from build123d import *

# Parameters (mm, degrees)
F2_R     = 7.5
F3_DEPTH = 40
F4_R     = 3
F5_DEPTH = 25


with BuildPart() as f1:
    # F0 (on Front) → F1 (revolve)
    with BuildSketch(Plane.XZ):
        Polygon((-78.328885, 0), (-47.328885, 0), (-47.328885, 19.231284), (-58.328885, 19.231284), (-58.328885, 17.231284), (-60.328885, 17.231284), (-60.328885, 19.231284), (-62.328885, 19.231284), (-62.328885, 17.231284), (-64.328885, 17.231284), (-64.328885, 19.231284), (-66.328885, 19.231284), (-66.328885, 17.231284), (-68.328885, 17.231284), (-68.328885, 19.231284), (-78.328885, 19.231284), align=None)
    revolve(axis=Axis((-39.164443, 0, 0), (-1, 0, 0)))

    # F2 (on face) → F3 (cut)
    with BuildSketch(Plane(origin=(-78.328885, 0, 0), x_dir=(0, -1, 0), z_dir=(-1, 0, 0))):
        Circle(F2_R)
    extrude(amount=-F3_DEPTH, mode=Mode.SUBTRACT)

    # F4 (on Top) → F5 (cut)
    with BuildSketch(Plane.XY):
        with Locations((-52.106317, 0)):
            Circle(F4_R)
    extrude(amount=F5_DEPTH, mode=Mode.SUBTRACT)


solid = f1.part
Design review of the part built by this model. Coordinates are the model's own, in mm. A direction names the side the tool comes from. Round coordinates to 2 decimals unless told otherwise and drop trailing zeros. Write each loop counter-clockwise with the first axis right and the second up, starting at its lowest first coordinate (ties: lowest second). Pieces come first, ordered by that corner, then holes. Notation, with made-up numbers: (17.5, 26.25) -> (37.5, 26.25) arc R9 ccw to (37.5, 32.25) -> close; hole circle Ø6 at (-2, 5.25). An arc over 180 degrees is marked (long way). One line per item, written item: value. Start each with the question number.
Q1. Add section D-D (x = -67). Give the boundary of the cut face in (y, z).
Q2. The part is to be moulded in two halves that separate along Y. For faces 1 (the face through (-61.343, -11.702, -15.261)), 2 (the face through (-49.245, 0.901, 12.966)), 3 (the face through (-66.329, 7, -16)), 4 (the face through (-63.05, 1.63, -7.32)), say which applies: pulls with the +Y half, pulls with the -Y half, needs draft (parallel to the pull), parting line crosses it, or undercut.
Q3. To check wall thickness, follow probe 1 along X at (y, z) = (0, 10); probe 2 along X at (y, z) = (-11, -15.5); probe 3 along Y at (x, z) = (-48.5, 6). State the ranges of each line that lie inside material, in increasing order.
Q4. Insertion check: P1, Ø12, axis at x = -72, y = 12.5, coming from the +Z side; P2, Ø6, axis at x = -68.5, z = -8, coming from the +Y side; P3, Ø12, axis at x = -74.5, z = 11, coming from the -Y side; P4, Ø17, axis at y = 0, z = 0, coming from the -X side. Each pin has a flat end and moves straight along its axis. Give the tip position at first contact, or say it passes through.
Q5. Tool access review of faces 5 (the face through (-73.399, -11.702, -15.261)), 6 (the face through (-62.329, 7, -16)): name each direction out of +Z, -Z, +X, -X, +Y, -Y from which nothing blocks a thin tool from reaching the whole face with its end or side.
Response:
1. outline: circle Ø34.46 at (0, 0); hole circle Ø15 at (0, 0)
2. face 1: parting line crosses it
2. face 2: undercut
2. face 3: needs draft
2. face 4: undercut
3. probe 1: x = -78.33 to -55.11, -49.11 to -47.33
3. probe 2: x = -78.33 to -68.33, -66.33 to -64.33, -62.33 to -60.33, -58.33 to -47.33
3. probe 3: y = -18.27 to -4.5, 4.5 to 18.27
4. P1: stops at z = 18.1
4. P2: stops at y = 18.57
4. P3: stops at y = -18.57
4. P4: stops at x = -78.33
5. face 5: +X, -X
5. face 6: none
